```python
from build123d import *

# Parameters (mm, degrees)
SKETCH_1_W          = 40
SKETCH_1_H          = 40
EXTRUDE_1_DEPTH     = 5
SKETCH_2_W          = 5
SKETCH_2_H          = 5
CUT_EXTRUDE_1_DEPTH = 1.8
SKETCH_4_W          = 5
SKETCH_4_H          = 5
CUT_EXTRUDE_2_DEPTH = 6.7
FILLET_1_R          = 3
HOLE_WIZARD_M2_1_D  = 2.4
FILLET_2_R          = 0.5
CUT_EXTRUDE_3_DEPTH = 4
SKETCH_7_R          = 13.5
CUT_EXTRUDE_4_DEPTH = 9
FILLET_3_R          = 1
SKETCH_9_R          = 12.5
EXTRUDE_2_DEPTH     = 9.5


with BuildPart() as part:
    # ｽｹｯﾁ1 → ﾎﾞｽ - 押し出し1 (new, symmetric)
    with BuildSketch(Plane(origin=(0, 0, 0), x_dir=(1, 0, 0), z_dir=(0, 1, 0))):
        Rectangle(SKETCH_1_W, SKETCH_1_H)
    extrude(amount=EXTRUDE_1_DEPTH, both=True)

    # ｽｹｯﾁ2 → ｶｯﾄ - 押し出し1 (cut)
    with BuildSketch(Plane(origin=(0, 5, 0), x_dir=(1, 0, 0), z_dir=(0, 1, 0))):
        with Locations((17.5, 17.5)):
            Rectangle(SKETCH_2_W, SKETCH_2_H)
        with Locations((-17.5, 17.5)):
            Rectangle(SKETCH_2_W, SKETCH_2_H)
        with Locations((-17.5, -17.5)):
            Rectangle(SKETCH_2_W, SKETCH_2_H)
        with Locations((17.5, -17.5)):
            Rectangle(SKETCH_2_W, SKETCH_2_H)
    extrude(amount=-CUT_EXTRUDE_1_DEPTH, mode=Mode.SUBTRACT)

    # ｽｹｯﾁ4 → ｶｯﾄ - 押し出し2 (cut)
    with BuildSketch(Plane.XZ.offset(5)):
        with Locations((17.5, -17.5)):
            Rectangle(SKETCH_4_W, SKETCH_4_H)
        with Locations((17.5, 17.5)):
            Rectangle(SKETCH_4_W, SKETCH_4_H)
        with Locations((-17.5, 17.5)):
            Rectangle(SKETCH_4_W, SKETCH_4_H)
        with Locations((-17.5, -17.5)):
            Rectangle(SKETCH_4_W, SKETCH_4_H)
    extrude(amount=-CUT_EXTRUDE_2_DEPTH, mode=Mode.SUBTRACT)

    # ﾌｨﾚｯﾄ1
    fillet_1_edges = [part.edges().sort_by_distance(p)[0] for p in [
        (-15, -1.65, -15),
        (20, 2.45, -20),
        (15, 4.1, -15),
        (-20, 2.45, -20),
        (20, 2.45, 20),
        (-20, 2.45, 20),
        (-15, 4.1, -15),
        (-15, 4.1, 15),
        (15, 4.1, 15),
        (15, -1.65, -15),
        (15, -1.65, 15),
        (-15, -1.65, 15),
    ]]
    fillet(fillet_1_edges, radius=FILLET_1_R)

    # M2 すきま穴1 (through all)
    with Locations(Plane(origin=(0, 3.2, 0), x_dir=(1, 0, 0), z_dir=(0, 1, 0))):
        with Locations((-17.5, -17.5), (-17.5, 17.5), (17.5, 17.5), (17.5, -17.5)):
            Hole(HOLE_WIZARD_M2_1_D / 2)

    # ﾌｨﾚｯﾄ2
    fillet_2_edges = [part.edges().sort_by_distance(p)[0] for p in [
        (-15, -1.65, -20),
        (-20, -1.65, -15),
        (20, 4.1, -15),
        (15, 4.1, -20),
        (-15, 4.1, -20),
        (-20, 4.1, -15),
        (-20, 4.1, 15),
        (-15, 4.1, 20),
        (15, 4.1, 20),
        (20, 4.1, 15),
        (20, -1.65, -15),
        (15, -1.65, -20),
        (15, -1.65, 20),
        (20, -1.65, 15),
        (-20, -1.65, 15),
        (-15, -1.65, 20),
    ]]
    fillet(fillet_2_edges, radius=FILLET_2_R)

    # ｽｹｯﾁ8 → ｶｯﾄ - 押し出し3 (cut, symmetric)
    with BuildSketch(Plane(origin=(0, 0, 0), x_dir=(1, 0, 0), z_dir=(0, 1, 0))):
        with BuildLine():
            Line((-14, 19), (-14, 20))
            Line((-14, 20), (14, 20))
            Line((14, 20), (14, 19))
            Line((14, 19), (14, 18))
            ThreePointArc((14, 18), (15.171572875, 15.171572875), (18, 14))
            Line((18, 14), (19, 14))
            Line((19, 14), (19, -14))
            Line((19, -14), (18, -14))
            ThreePointArc((18, -14), (15.171572875, -15.171572875), (14, -18))
            Line((14, -18), (14, -19))
            Line((14, -19), (-14, -19))
            Line((-14, -19), (-14, -18))
            ThreePointArc((-14, -18), (-15.171572875, -15.171572875), (-18, -14))
            Line((-18, -14), (-19, -14))
            Line((-19, -14), (-19, 14))
            Line((-19, 14), (-18, 14))
            ThreePointArc((-18, 14), (-15.171572875, 15.171572875), (-14, 18))
            Line((-14, 18), (-14, 19))
        make_face()
    extrude(amount=CUT_EXTRUDE_3_DEPTH, both=True, mode=Mode.SUBTRACT)

    # ｽｹｯﾁ7 → ｶｯﾄ - 押し出し4 (cut)
    with BuildSketch(Plane.XZ.offset(-5)):
        with Locations(Location((-3.5, 0, 0), (0, 0, 90))):
            Circle(SKETCH_7_R)
    extrude(amount=CUT_EXTRUDE_4_DEPTH, mode=Mode.SUBTRACT)

    # ﾌｨﾚｯﾄ3
    fillet_3_edges = [part.edges().sort_by_distance(p)[0] for p in [
        (-3.5, 5, -13.5),
    ]]
    fillet(fillet_3_edges, radius=FILLET_3_R - 0.0001)  # a hair under: the kernel refuses the full size

    # ｽｹｯﾁ9 → ﾎﾞｽ - 押し出し2 (add)
    with BuildSketch(Plane(origin=(0, -4, 0), x_dir=(1, 0, 0), z_dir=(0, 1, 0))):
        with Locations(Location((-3.5, 0, 0), (0, 0, 270))):
            Circle(SKETCH_9_R)
    extrude(amount=EXTRUDE_2_DEPTH)


solid = part.part
```
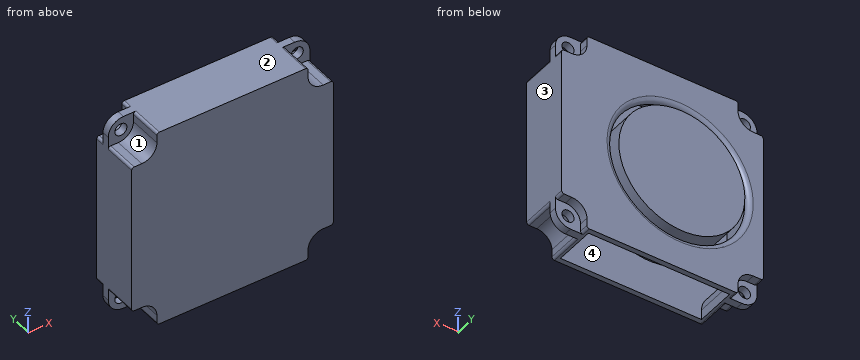
Geometry: final body of the model. Coordinates: model frame, mm. Face numbers are marked on the shaded views. Round coordinates to 2 decimals unless told otherwise and drop trailing zeros. Order: outer loops, then holes, each group sorted by start corner. A loop starts at its lowest first (then second) coordinate and runs counter-clockwise, first axis right, second up. Notation, with made-up numbers: (71.25, 11) -> (86.25, 11) arc R32 ccw to (86.25, 47) -> close; hole circle Ø2 at (-36.5, 80). An arc over 180 degrees is marked (long way). Use one line per item in the form item = value.
(1) Ray query, probe 1 along Y at (x, z) = (13.5, 2); probe 2 along X at (y, z) = (4.05, 0); probe 3 along X at (y, z) = (2.75, 17.5). Return the intervals inside material, ascending. Write a range as [from, to].
Results list:
probe_1 = [-5, -4], [4, 5]
probe_2 = [-20, -17], [-16, 9], [10, 20]
probe_3 = [-19.96, -18.7], [-16.3, -14.03], [14.03, 16.3], [18.7, 19.96]
(2) Section A-A on y = 4.5. Return loops of the section in (x, z).
Results list:
outline = (-20, -14.5) arc R0.5 ccw to (-19.5, -15) -> (-18, -15) arc R3 cw to (-15, -18) -> (-15, -19.5) arc R0.5 ccw to (-14.5, -20) -> (14.5, -20) arc R0.5 ccw to (15, -19.5) -> (15, -18) arc R3 cw to (18, -15) -> (19.5, -15) arc R0.5 ccw to (20, -14.5) -> (20, 14.5) arc R0.5 ccw to (19.5, 15) -> (18, 15) arc R3 cw to (15, 18) -> (15, 19.5) arc R0.5 ccw to (14.5, 20) -> (-14.5, 20) arc R0.5 ccw to (-15, 19.5) -> (-15, 18) arc R3 cw to (-18, 15) -> (-19.5, 15) arc R0.5 ccw to (-20, 14.5) -> close; circle Ø25 at (-3.5, 0); hole circle Ø27.27 at (-3.5, 0)
(3) Section C-C on x = 17.5. Return loops of the section in (y, z).
Results list:
outline = (-5, -15.04) -> (1.7, -15.04) -> (1.7, -16.3) -> (3.2, -16.3) -> (3.2, -15.04) -> (5, -15.04) -> (5, 15.04) -> (3.2, 15.04) -> (3.2, 16.3) -> (1.7, 16.3) -> (1.7, 15.04) -> (-5, 15.04) -> close; (1.7, -19.96) -> (3.2, -19.96) -> (3.2, -18.7) -> (1.7, -18.7) -> close; (1.7, 18.7) -> (3.2, 18.7) -> (3.2, 19.96) -> (1.7, 19.96) -> close; hole (-4, -14.03) -> (4, -14.03) -> (4, 14.03) -> (-4, 14.03) -> close
(4) Draft query along X for the marked faces 1, 2, 3 and 4. Return one class per face: pulls with the +X half, pulls with the -X half, needs draft (parallel to the pull), parting line crosses it, or undercut.
Results list:
face_1 = pulls with the -X half
face_2 = needs draft
face_3 = pulls with the +X half
face_4 = undercut
(5) First-contact query: pin 1 Ø0.6 at (y, z) = (-0.5, -19.5) entering from -X; pin 2 Ø3 at (x, z) = (17.5, 18) entering from +Y; pin 3 Ø3 at (x, z) = (-17.5, 17.5) entering from -Y. Flat tips, straight axial feed; report the tip coordinate or a pass-through.
Results list:
pin_1 = -15
pin_2 = 3.2
pin_3 = 1.7
